Source: three-view drawing plus pictorial views. Frame: mm from the lowest corner of the part. Coordinates: 2 decimals unless noted, no trailing zeros. Write each loop counter-clockwise with the first axis right and the second up, starting at its lowest first coordinate (ties: lowest second). Pieces come first, ordered by that corner, then holes.
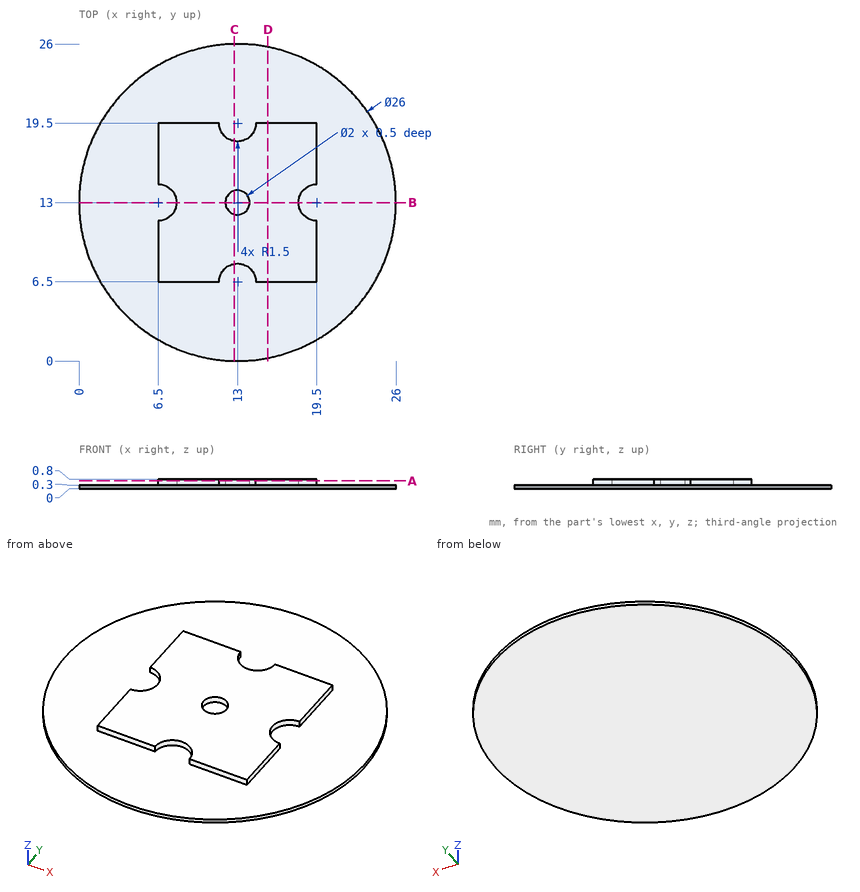
Item 1: Section query A-A, the plane z = 0.65. Return loops of the section in (x, y), then the cut area to 3 significant figures.
Item 2: Section query D-D, the plane x = 15.5. Return loops of the section in (y, z), then the cut area to 3 significant figures.
Item 3: Section query C-C, the plane x = 12.75. Return loops of the section in (y, z), then the cut area to 3 significant figures.
Item 4: Material intervals for line 1 (Y direction, x = 13, z = 0.7); line 2 (Z direction, x = 20.5, y = 15.25); line 3 (X direction, y = 11, z = 0.75), sorted ascending.
Item 5: Section query B-B, the plane y = 13. Return loops of the section in (x, z), then the cut area to 3 significant figures.
Item 6: Pin query (flat end, axial travel): pin 1 Ø3 at (x, y) = (4.5, 4.5) entering from +Z. Return the tip coordinate at first contact, or that it passes through.
The answers:
1. outline: (6.5, 6.5) - (11.5, 6.5) arc R1.5 cw to (14.5, 6.5) - (19.5, 6.5) - (19.5, 11.5) arc R1.5 cw to (19.5, 14.5) - (19.5, 19.5) - (14.5, 19.5) arc R1.5 cw to (11.5, 19.5) - (6.5, 19.5) - (6.5, 14.5) arc R1.5 cw to (6.5, 11.5) - close; hole circle Ø2 at (13, 13)
1. area: 152 mm2
2. outline: (0.24, 0) - (25.76, 0) - (25.76, 0.3) - (19.5, 0.3) - (19.5, 0.8) - (6.5, 0.8) - (6.5, 0.3) - (0.24, 0.3) - close
2. area: 14.2 mm2
3. outline: (0, 0) - (26, 0) - (26, 0.3) - (18.02, 0.3) - (18.02, 0.8) - (13.97, 0.8) - (13.97, 0.3) - (12.03, 0.3) - (12.03, 0.8) - (7.98, 0.8) - (7.98, 0.3) - (0, 0.3) - close
3. area: 11.9 mm2
4. line 1: y = 8 to 12, 14 to 18
4. line 2: z = 0 to 0.3
4. line 3: x = 6.5 to 19.5
5. outline: (0, 0) - (26, 0) - (26, 0.3) - (18, 0.3) - (18, 0.8) - (14, 0.8) - (14, 0.3) - (12, 0.3) - (12, 0.8) - (8, 0.8) - (8, 0.3) - (0, 0.3) - close
5. area: 11.8 mm2
6. pin 1: stops at z = 0.3
